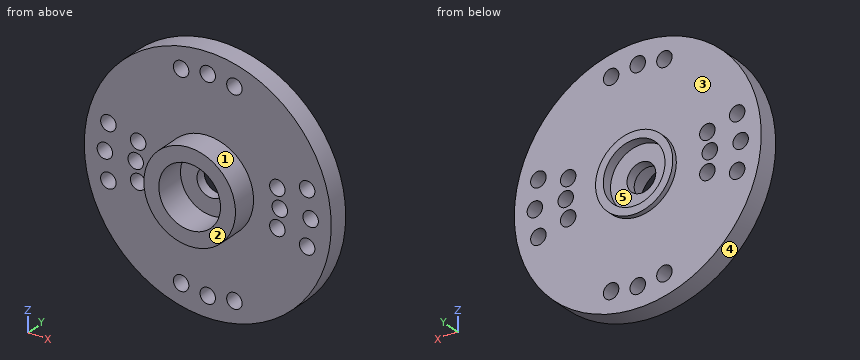
from build123d import *

# Parameters (mm, degrees)
F_1_5_1_5_DIAMETER_HOLE1_D     = 1.5
F_1_5_1_5_DIAMETER_HOLE1_DEPTH = 2
CIRPATTERN1_COUNT              = 4
SKETCH4_R                      = 3
CUT_EXTRUDE1_DEPTH             = 1
SKETCH5_R                      = 3
CUT_EXTRUDE2_DEPTH             = 3
F_1_5_1_5_DIAMETER_HOLE2_D     = 1.5
F_1_5_1_5_DIAMETER_HOLE2_DEPTH = 2
CIRPATTERN2_COUNT              = 2


with BuildPart() as part:
    # Sketch1 → Revolve1 (revolve)
    with BuildSketch(Plane.XY):
        Polygon((-12, 0), (-3.75, 0), (-3.75, 0.5), (-1.4, 0.5), (-1.4, -4.5), (-4.45, -4.5), (-4.45, -2), (-12, -2), align=None)
    revolve(axis=Axis((0, 0, 0), (0, -1, 0)))

    # Ø1.5 (1.5) Diameter Hole1
    with Locations(Plane(origin=(0, 0, 0), x_dir=(-1, 0, 0), z_dir=(0, 1, 0))):
        with Locations((0, -10), (2.588190451, -9.659258263), (-2.588190451, -9.659258263)):
            f_1_5_1_5_diameter_hole1 = Hole(F_1_5_1_5_DIAMETER_HOLE1_D / 2, depth=F_1_5_1_5_DIAMETER_HOLE1_DEPTH)

    # CirPattern1: Ø1.5 (1.5) Diameter Hole1 ×4 about axis
    cirpattern1_axis = Axis((0, 0, 0), (0, 1, 0))
    for i in range(1, CIRPATTERN1_COUNT):
        add(f_1_5_1_5_diameter_hole1.rotate(cirpattern1_axis, i * 360 / CIRPATTERN1_COUNT), mode=Mode.SUBTRACT)

    # Sketch4 → Cut-Extrude1 (cut)
    with BuildSketch(Plane(origin=(0, 0.5, 0), x_dir=(-1, 0, 0), z_dir=(0, 1, 0))):
        Circle(SKETCH4_R)
    extrude(amount=-CUT_EXTRUDE1_DEPTH, mode=Mode.SUBTRACT)

    # Sketch5 → Cut-Extrude2 (cut)
    with BuildSketch(Plane.XZ.offset(4.5)):
        Circle(SKETCH5_R)
    extrude(amount=-CUT_EXTRUDE2_DEPTH, mode=Mode.SUBTRACT)

    # Ø1.5 (1.5) Diameter Hole2
    with Locations(Plane(origin=(0, 0, 0), x_dir=(-1, 0, 0), z_dir=(0, 1, 0))):
        with Locations((6.761480784, -1.811733316), (7, 0), (6.761480784, 1.811733316)):
            f_1_5_1_5_diameter_hole2 = Hole(F_1_5_1_5_DIAMETER_HOLE2_D / 2, depth=F_1_5_1_5_DIAMETER_HOLE2_DEPTH)

    # CirPattern2: Ø1.5 (1.5) Diameter Hole2 ×2 about axis
    cirpattern2_axis = Axis((0, 0, 0), (0, 1, 0))
    for i in range(1, CIRPATTERN2_COUNT):
        add(f_1_5_1_5_diameter_hole2.rotate(cirpattern2_axis, i * 360 / CIRPATTERN2_COUNT), mode=Mode.SUBTRACT)


solid = part.part
Can you work these out from the model? Positions are in its coordinate system, mm. Face numbers are marked on the shaded views. A direction names the side the tool comes from. Coordinates: 2 decimals unless noted, no trailing zeros. Write each loop counter-clockwise with the first axis right and the second up, starting at its lowest first coordinate (ties: lowest second). Pieces come first, ordered by that corner, then holes. Notation, with made-up numbers: (-10.5, -5.5) -> (20.5, -5.5) arc R29 ccw to (20.5, 27.5) -> close; hole circle Ø6 at (-28.75, -26.5). An arc over 180 degrees is marked (long way). Write item = value, one per line.
(1) Imagine slicing it at D-D (y = -4.1). Please give me the cut outline in (x, z).
Verdict:
outline = circle Ø8.9 at (0, 0); hole circle Ø6 at (0, 0)
(2) Imagine slicing it at A-A (x = 0). State how many separate pieces and enclosed holes the cut face has, and give its area (3 significant figures).
Verdict:
separate_pieces = 4
enclosed_holes = 0
area = 41.2 mm^2
(3) If I drill on probe 1 along Z at (x, y) = (2.5, -1.4); probe 2 along Z at (x, y) = (-2, -0.45); probe 3 along Z at (x, y) = (0, -3.75), over which ranges is the centre line in solid material (lowest first)?
Verdict:
probe_1 = -11.74 to -10.4, -8.91 to 8.91, 10.4 to 11.74
probe_2 = -11.83 to -10.12, -9.19 to -2.24, 2.24 to 9.19, 10.12 to 11.83
probe_3 = -4.45 to -3, 3 to 4.45
(4) Imagine slicing it at C-C (x = -2.5). Please give me the cut outline in (y, z), and give its area (3 significant figures).
Verdict:
outline = (-4.5, -3.68) -> (-2, -3.68) -> (-2, -8.91) -> (0, -8.91) -> (0, -2.8) -> (0.5, -2.8) -> (0.5, -1.66) -> (-0.5, -1.66) -> (-0.5, 1.66) -> (0.5, 1.66) -> (0.5, 2.8) -> (0, 2.8) -> (0, 8.91) -> (-2, 8.91) -> (-2, 3.68) -> (-4.5, 3.68) -> (-4.5, 1.66) -> (-1.5, 1.66) -> (-1.5, -1.66) -> (-4.5, -1.66) -> close; (-2, -11.74) -> (0, -11.74) -> (0, -10.4) -> (-2, -10.4) -> close; (-2, 10.4) -> (0, 10.4) -> (0, 11.74) -> (-2, 11.74) -> close
area = 48.9 mm^2
(5) Imagine slicing it at B-B (z = 10). Please give me the cut outline in (x, y), and give its area (3 significant figures).
Verdict:
outline = (-6.63, -2) -> (-3.26, -2) -> (-3.26, 0) -> (-6.63, 0) -> close; (-1.92, -2) -> (-0.75, -2) -> (-0.75, 0) -> (-1.92, 0) -> close; (0.75, -2) -> (1.92, -2) -> (1.92, 0) -> (0.75, 0) -> close; (3.26, -2) -> (6.63, -2) -> (6.63, 0) -> (3.26, 0) -> close
area = 18.2 mm^2
(6) On a 3-axis mill with a long thin cutter (end or side, diameter ignored), from which of +Z, -Z, +X, -X, +Y, -Y can I reach the whole of each face in a straight line? I mean the marked faces 1 and 2. Say none if no direction works.
Verdict:
face_1 = -Y
face_2 = +Z, -Z, +X, -X, -Y
(7) Thinking about a two-plate mould opening in X: for the marked faces 3, 4 and 5, which applies, +X half, -X half, draft (parallel to the pull), parting line (faces both ways), or undercut?
Verdict:
face_3 = draft
face_4 = parting line
face_5 = undercut
(8) For pin 1 (1.2 mm diameter, centred on x = -10, z = 0, fed in from +Y); pin 2 (2 mm diameter, centred on x = 0, z = -10, fed in from +Y); pin 3 (6 mm diameter, centred on x = -7, z = -3, fed in from -Y); pin 4 (2 mm diameter, centred on y = -2.5, z = -4.5, fed in from +X), each with a flat end and sliding along its axis, tell me the tip position at first contact or that it passes through.
Verdict:
pin_1 = through
pin_2 = 0
pin_3 = -2
pin_4 = 11.44
